Build history of the part. All positions in model axes, mm. A direction names the side the tool comes from. Coordinates: 2 decimals unless noted, no trailing zeros. Loops run counter-clockwise (first coordinate to the right, second up) from the corner with the lowest first, then second, coordinate; pieces in that order, holes last.
(1) Wall check: L1, parallel to Z at x = 74.5, y = 37.5; L2, parallel to Y at x = 53.85, z = -61; L3, parallel to Y at x = 69.85, z = -2.5. Give the ranges that are in metal, low to high.
(2) Slice it at B-B (x = 24). Give the cut face in (y, z), and give its area (3 significant figures).
(3) Slice it at A-A (y = 40). Give the cut face in (x, z).
(4) Two-plate mould, pull along X, no slides. Class faces 5 (the face through (50, 50.8, -60)), 6 (the face through (88.1, 31.8, -60.4)), 7 (the face through (5.43, 5.73, -3.22)): pulls with the +X half, pulls with the -X half, needs draft (parallel to the pull), parting line crosses it, or undercut.
(5) Slice it at C-C (x = 53.85). Give the cut face in (y, z).
(6) Flat gauge pins, fed straight in: P1, Ø10, axis at x = 85, z = -30, coming from the +Y side; P2, Ø4.5, axis at x = 95.6, y = 44.8, coming from the -Z side; P3, Ø6, axis at x = 81, y = 7, coming from the -Z side; P4, Ø12, axis at x = 81, z = -16.5, coming from the -Y side. Where does each tip first touch, or does it go through?
(7) Tool access for faces 1 (the face through (14.61, 22.18, -55.34)), 2 (the face through (89, 25.4, -31)), 3 (the face through (50, 35, -63.5)), 4 (the face through (63, 19.05, -60)): list every direction of +Z, -Z, +X, -X, +Y, -Y with a clear straight run to the whole face (end or side of a thin tool).
(8) Slice it at D-D (y = 31.75). Give the cut face in (x, z).
from build123d import *

# Parameters (mm, degrees)
SKETCH1_W           = 101.6
SKETCH1_H           = 63.5
BOSS_EXTRUDE1_DEPTH = 50.8
CUT_EXTRUDE1_REACH  = 132.136
SKETCH2_W           = 50.8
SKETCH2_H           = 25.4
SKETCH2_W_2         = 57.15
SKETCH2_H_2         = 19.05
SKETCH5_W           = 63.5
SKETCH5_H           = 50.8
CUT_EXTRUDE5_DEPTH  = 6.35
CUT_EXTRUDE2_REACH  = 132.136
SKETCH3_R           = 2.25
CUT_EXTRUDE3_REACH  = 132.136
CUT_EXTRUDE4_REACH  = 132.136
SKETCH4_R           = 2.54
FILLET1_R           = 19.05
FILLET2_R           = 6.35


with BuildPart() as part:
    # Sketch1 → Boss-Extrude1 (new body)
    with BuildSketch(Plane(origin=(0, 0, 0), x_dir=(1, 0, 0), z_dir=(0, 1, 0))):
        with Locations((50.8, 31.75)):
            Rectangle(SKETCH1_W, SKETCH1_H)
    extrude(amount=BOSS_EXTRUDE1_DEPTH)

    # Sketch2 → Cut-Extrude1 (cut, up to next)
    with BuildSketch(Plane(origin=(101.6, 0, 0), x_dir=(0, 0, -1), z_dir=(1, 0, 0)), mode=Mode.PRIVATE) as cut_extrude1_sk1:
        with Locations((31.75, 38.1)):
            Rectangle(SKETCH2_W, SKETCH2_H)
    cut_extrude1_tool1 = extrude(cut_extrude1_sk1.sketch, amount=-CUT_EXTRUDE1_REACH, mode=Mode.PRIVATE) & part.part
    # Sketch2 → Cut-Extrude1 (cut, up to next)
    with BuildSketch(Plane(origin=(101.6, 0, 0), x_dir=(0, 0, -1), z_dir=(1, 0, 0)), mode=Mode.PRIVATE) as cut_extrude1_sk2:
        with Locations((34.925, 9.525)):
            Rectangle(SKETCH2_W_2, SKETCH2_H_2)
    cut_extrude1_tool2 = extrude(cut_extrude1_sk2.sketch, amount=-CUT_EXTRUDE1_REACH, mode=Mode.PRIVATE) & part.part
    add(cut_extrude1_tool1.solids().sort_by_distance((101.6, 38.1, -31.75))[0], mode=Mode.SUBTRACT)
    add(cut_extrude1_tool2.solids().sort_by_distance((101.6, 9.525, -34.925))[0], mode=Mode.SUBTRACT)

    # Sketch5 → Cut-Extrude5 (cut)
    with BuildSketch(Plane(origin=(0, 25.4, 0), x_dir=(1, 0, 0), z_dir=(0, 1, 0))):
        with Locations((44.45, 31.75)):
            Rectangle(SKETCH5_W, SKETCH5_H)
    extrude(amount=-CUT_EXTRUDE5_DEPTH, mode=Mode.SUBTRACT)

    # Sketch3 → Cut-Extrude2 (cut, up to next)
    with BuildSketch(Plane(origin=(0, 0, -63.5), x_dir=(-1, 0, 0), z_dir=(0, 0, -1)), mode=Mode.PRIVATE) as cut_extrude2_sk1:
        with Locations((-85.85, 31.75)):
            Circle(SKETCH3_R)
    cut_extrude2_tool1 = extrude(cut_extrude2_sk1.sketch, amount=-CUT_EXTRUDE2_REACH, mode=Mode.PRIVATE) & part.part
    # Sketch3 → Cut-Extrude2 (cut, up to next)
    with BuildSketch(Plane(origin=(0, 0, -63.5), x_dir=(-1, 0, 0), z_dir=(0, 0, -1)), mode=Mode.PRIVATE) as cut_extrude2_sk2:
        with Locations((-53.85, 31.75)):
            Circle(SKETCH3_R)
    cut_extrude2_tool2 = extrude(cut_extrude2_sk2.sketch, amount=-CUT_EXTRUDE2_REACH, mode=Mode.PRIVATE) & part.part
    add(cut_extrude2_tool1.solids().sort_by_distance((85.85, 31.75, -63.5))[0], mode=Mode.SUBTRACT)
    add(cut_extrude2_tool2.solids().sort_by_distance((53.85, 31.75, -63.5))[0], mode=Mode.SUBTRACT)

    # Cut-Extrude3: up to this face of the body (flat: up to its plane)
    cut_extrude3_end = Plane(part.part.faces().sort_by_distance((50.8, 25.4, 0))[0])
    # Sketch3<4> → Cut-Extrude3 (cut, up to the picked face)
    with BuildSketch(Plane(origin=(0, 0, -63.5), x_dir=(-1, 0, 0), z_dir=(0, 0, -1)), mode=Mode.PRIVATE) as cut_extrude3_sk1:
        with BuildLine():
            ThreePointArc((-65.05, 31.75), (-69.85, 36.55), (-74.65, 31.75))
            Line((-74.65, 31.75), (-65.05, 31.75))
        make_face()
    cut_extrude3_tool1 = split(extrude(cut_extrude3_sk1.sketch, amount=-CUT_EXTRUDE3_REACH, mode=Mode.PRIVATE), bisect_by=cut_extrude3_end, keep=Keep.BOTH, mode=Mode.PRIVATE)
    # Sketch3<4> → Cut-Extrude3 (cut, up to the picked face)
    with BuildSketch(Plane(origin=(0, 0, -63.5), x_dir=(-1, 0, 0), z_dir=(0, 0, -1)), mode=Mode.PRIVATE) as cut_extrude3_sk2:
        with BuildLine():
            Line((-65.05, 31.75), (-74.65, 31.75))
            ThreePointArc((-74.65, 31.75), (-69.85, 26.95), (-65.05, 31.75))
        make_face()
    cut_extrude3_tool2 = split(extrude(cut_extrude3_sk2.sketch, amount=-CUT_EXTRUDE3_REACH, mode=Mode.PRIVATE), bisect_by=cut_extrude3_end, keep=Keep.BOTH, mode=Mode.PRIVATE)
    # Sketch3<4> → Cut-Extrude3 (cut, up to the picked face)
    with BuildSketch(Plane(origin=(0, 0, -63.5), x_dir=(-1, 0, 0), z_dir=(0, 0, -1)), mode=Mode.PRIVATE) as cut_extrude3_sk3:
        with BuildLine():
            ThreePointArc((-65.05, 31.75), (-69.85, 36.55), (-74.65, 31.75))
            Line((-74.65, 31.75), (-65.05, 31.75))
        make_face()
    cut_extrude3_tool3 = split(extrude(cut_extrude3_sk3.sketch, amount=-CUT_EXTRUDE3_REACH, mode=Mode.PRIVATE), bisect_by=cut_extrude3_end, keep=Keep.BOTH, mode=Mode.PRIVATE)
    # Sketch3<4> → Cut-Extrude3 (cut, up to the picked face)
    with BuildSketch(Plane(origin=(0, 0, -63.5), x_dir=(-1, 0, 0), z_dir=(0, 0, -1)), mode=Mode.PRIVATE) as cut_extrude3_sk4:
        with BuildLine():
            Line((-65.05, 31.75), (-74.65, 31.75))
            ThreePointArc((-74.65, 31.75), (-69.85, 26.95), (-65.05, 31.75))
        make_face()
    cut_extrude3_tool4 = split(extrude(cut_extrude3_sk4.sketch, amount=-CUT_EXTRUDE3_REACH, mode=Mode.PRIVATE), bisect_by=cut_extrude3_end, keep=Keep.BOTH, mode=Mode.PRIVATE)
    add(cut_extrude3_tool1.solids().sort_by(Axis((69.85, 33.787183, -63.5), (0, 0, 1)))[0], mode=Mode.SUBTRACT)
    add(cut_extrude3_tool2.solids().sort_by(Axis((69.85, 29.712817, -63.5), (0, 0, 1)))[0], mode=Mode.SUBTRACT)
    add(cut_extrude3_tool3.solids().sort_by(Axis((69.85, 33.787183, -63.5), (0, 0, 1)))[0], mode=Mode.SUBTRACT)
    add(cut_extrude3_tool4.solids().sort_by(Axis((69.85, 29.712817, -63.5), (0, 0, 1)))[0], mode=Mode.SUBTRACT)

    # Cut-Extrude4: up to this face of the body (flat: up to its plane)
    cut_extrude4_end = Plane(part.part.faces().sort_by_distance((50.529040984, 25.309680328, 0))[0])
    # Sketch4 → Cut-Extrude4 (cut, up to the picked face)
    with BuildSketch(Plane(origin=(0, 0, -63.5), x_dir=(-1, 0, 0), z_dir=(0, 0, -1)), mode=Mode.PRIVATE) as cut_extrude4_sk1:
        with Locations((-95.6, 44.8)):
            Circle(SKETCH4_R)
    cut_extrude4_tool1 = split(extrude(cut_extrude4_sk1.sketch, amount=-CUT_EXTRUDE4_REACH, mode=Mode.PRIVATE), bisect_by=cut_extrude4_end, keep=Keep.BOTH, mode=Mode.PRIVATE)
    add(cut_extrude4_tool1.solids().sort_by(Axis((95.6, 44.8, -63.5), (0, 0, 1)))[0], mode=Mode.SUBTRACT)

    # Fillet1
    fillet1_edges = [part.edges().sort_by_distance(p)[0] for p in [
        (0, 0, -3.175),
        (101.6, 0, -3.175),
    ]]
    fillet(fillet1_edges, radius=FILLET1_R)

    # Fillet2
    fillet2_edges = [part.edges().sort_by_distance(p)[0] for p in [
        (12.7, 22.225, -6.35),
        (12.7, 22.225, -57.15),
        (76.2, 22.225, -57.15),
        (76.2, 22.225, -6.35),
    ]]
    fillet(fillet2_edges, radius=FILLET2_R)


solid = part.part
Response values:
1. L1: z = -63.5 to -57.15, -6.35 to 0
1. L2: y = 19.05 to 29.5, 34 to 50.8
1. L3: y = 0 to 26.95, 36.55 to 50.8
2. outline: (0, -6.35) - (50.8, -6.35) - (50.8, 0) - (0, 0) - close; (19.05, -63.5) - (50.8, -63.5) - (50.8, -57.15) - (19.05, -57.15) - close
2. area: 524 mm2
3. outline: (0, -63.5) - (101.6, -63.5) - (101.6, -57.15) - (0, -57.15) - close; (0, -6.35) - (101.6, -6.35) - (101.6, 0) - (0, 0) - close
4. face 5: needs draft
4. face 6: undercut
4. face 7: pulls with the -X half
5. outline: (0, -6.35) - (50.8, -6.35) - (50.8, 0) - (0, 0) - close; (19.05, -63.5) - (29.5, -63.5) - (29.5, -57.15) - (19.05, -57.15) - close; (34, -63.5) - (50.8, -63.5) - (50.8, -57.15) - (34, -57.15) - close
6. P1: stops at y = 25.4
6. P2: passes through
6. P3: stops at z = -6.35
6. P4: stops at y = 19.05
7. face 1: +Y, -Y
7. face 2: +X, -X, +Y
7. face 3: -Z, +X, -X, +Y, -Y
7. face 4: -Z, +X, -X, -Y
8. outline: (0, -63.5) - (51.6, -63.5) - (51.6, -57.15) - (0, -57.15) - close; (0, -6.35) - (65.05, -6.35) - (65.05, 0) - (0, 0) - close; (56.1, -63.5) - (65.05, -63.5) - (65.05, -57.15) - (56.1, -57.15) - close; (74.65, -63.5) - (83.6, -63.5) - (83.6, -57.15) - (74.65, -57.15) - close; (74.65, -6.35) - (101.6, -6.35) - (101.6, 0) - (74.65, 0) - close; (88.1, -63.5) - (101.6, -63.5) - (101.6, -57.15) - (88.1, -57.15) - close
